Autodesk Inventor part; units mm, degrees
ref_plane "Work Plane1" through (29, 0, 0) normal (0, -1, 0) x (1, 0, 0)
ref_plane "YZ Plane" through (0, 0, 0) normal (1, 0, 0) x (0, 1, 0)
ref_plane "XZ Plane" through (0, 0, 0) normal (0, 1, 0) x (-1, 0, 0)
sketch "Sketch1" plane through (0, 0, 0) normal (0, 0, 1) x (1, 0, 0)
  line L0 (0.2, 0) -> (20, 0)
  line L1 (20, 0) -> (20, 2.5)
  line L2 (20, 2.5) -> (2.4, 2.5)
  line L3 (2.4, 2.5) -> (1.9091, 2.5)
  line L4 (1.9091, 2.5) -> (0, 2.5)
  line L5 (0, 2.5) -> (0, 4.25)
  line L6 (0, 4.25) -> (-3.5, 4.25)
  line L7 (-3.5, 4.25) -> (-3.5, 1.7321)
  line L8 (-3.5, 1.7321) -> (-0.8, 1.7321)
  line L9 (-0.8, 1.7321) -> (0.2, 0)
  line L10 (-8.2, 0) -> (24.7, 0)
  line L11 (0, -0.85) -> (0, 5.1)
  line L12 (2.4, 2.5) -> (0, 2.5) construction
  dimension "d1" = 17.6
  dimension "d2" = 0.4909
  dimension "d3" = 3.5
  dimension "d4" = 2.7
  dimension "d5" = 60
  dimension "d6" = 5
  dimension "d7" = 5
  dimension "d8" = 3.4641
  dimension "d9" = 8.5
  dimension "d26" = 20
revolve "Body" add sketch "Sketch1" angle 360 about axis through (0.2, 0, 0) along (1, 0, 0) contours L9 L11 L4 L3 L2 L1 L0 | L9 L8 L7 L6 L5 L11
sketch "Sketch2" plane through (-3.5, 0, 0) normal (-1, 0, 0) x (0, 0, 1)
  circle A0 centre (0, 0) radius 1.7321
  line L0 (0, -5.95) -> (0, 5.95)
  line L1 (-5.95, 0) -> (5.95, 0)
  line L2 (1.7321, 0) -> (0.866, -1.5)
  line L3 (0.866, -1.5) -> (-0.866, -1.5)
  line L4 (-0.866, -1.5) -> (-1.7321, 0)
  line L5 (-1.7321, 0) -> (-0.866, 1.5)
  line L6 (-0.866, 1.5) -> (0.866, 1.5)
  line L7 (0.866, 1.5) -> (1.7321, 0)
extrude "Slot" add sketch "Sketch2" against normal up to next contours L7 A0 | A0 L2 | L6 L0 A0 | A0 L0 L3 | L0 L6 A0 | A0 L3 L0 | L4 A0 | A0 L5
fillet "Fillet1" radius 0.5 1 edges at (-3.5, -4.25, 0)
thread "Thread"
chamfer "Chamfer1" distance 0.4908 distance2 0.4908 1 edges at (20, -2.5, 0) measured on face at (20, -0.7379, -0.3873)
ref_plane "Work Plane1" through (29, 0, 0) normal (0, -1, 0) x (1, 0, 0)
fillet "Fillet2" radius 0.1 1 edges at (0, -2.5, 0)
equation "\"d1\" = GEL"
equation "\"d3\" = KOH"
equation "\"d4\" = INTI"
equation "\"d6\" = GD"
equation "\"d7\" = BDM"
equation "\"d8\" = 1.1547 * SW"
equation "\"d9\" = KOD"
equation "\"d26\" = NLG"
equation "\"d30\" = R"
equation "\"d17\" = RR"
equation "\"d13\" = GEL"
equation "\"d15\" = -0.5 * SPD + 0.5 * GD"
equation "\"d16\" = GUL"
equation "\"GD\" = NND"
equation "\"NLG\" = 20"
equation "\"GEL\" = 17.6"
equation "\"KOD\" = 8.5"
equation "\"KOH\" = 3.5"
equation "\"INTI\" = 2.7"
equation "\"GAL\" = 0.61345 * PTC"
equation "\"GUL\" = 0.61345 * PTC"
equation "\"BDM\" = NND"
equation "\"SW\" = 3"
equation "\"RR\" = 0.5"
equation "\"SPD\" = NND - 1.2269 * PTC"
equation "\"R\" = 0.1"
equation "\"TOA\" = 30deg"
equation "\"GD1\" = THREADDIA - 1.2269 * PTC"
equation "\"THREADDIA\" = 5"
equation "\"FAWI\" = 45deg"
equation "\"ANG\" = 120deg"
equation "\"PTC\" = 0.8"
equation "\"NND\" = 5"
equation "\"E0\" = 1.155 * SW"
properties part number "DIN 7984 - M5 x 20" material "Steel, Mild"
CAD build for the part. Positions are in the model's coordinates, mm. A direction names the side the tool comes from. Coordinates: 2 decimals unless noted, no trailing zeros. Write each loop counter-clockwise with the first axis right and the second up, starting at its lowest first coordinate (ties: lowest second). Pieces come first, ordered by that corner, then holes. Notation, with made-up numbers: (66.5, 46.5) -> (104.5, 46.5) arc R17 ccw to (104.5, 74.5) -> close; hole circle Ø7 at (-29.75, -24.75). An arc over 180 degrees is marked (long way). Return JSON: item names as keys, results as strings. Group by question number.
Q1. Pull direction Z, two halves, no side cores. Call faces 4 (the face through (20, 0, 0)), 5 (the face through (-1.521, 2.285, -3.584)), 6 (the face through (-2, 1.5, 0)): released by +Z, released by -Z, zero draft, split by the parting line, or undercut.
Q2. Flat gauge pins, fed straight in: pin 1 (4 mm diameter, centred on x = 16.5, z = -3, fed in from +Y); pin 2 (4 mm diameter, centred on x = 6.5, z = -3.5, fed in from -Y); pin 3 (5 mm diameter, centred on x = 3, y = -3, fed in from +Z). Where does each tip first touch, or does it go through?
Q3. Which spindle directions (+Z, -Z, +X, -X, +Y, -Y) get a long thin tool onto all of the face, cutting with end or side? Do faces 1 (the face through (0, 2, 2)), 2 (the face through (-3.5, -2, 0)), 3 (the face through (-2, -1.5, 0)). Say none if no direction does.
Q4. Drill centre lines: line 1 (X direction, y = 2.25, z = -2.75); line 2 (Z direction, x = -1.5, y = 1.25); line 3 (Z direction, x = 5, y = 2). Where is each one in solid material? Low to high.
Q5. Cut at A-A, the plane x = 9.5. Give the cut face in (y, z), then the cut area to 3 significant figures.
Returned:
{
 "1": {"face 4": "zero draft", "face 5": "split by the parting line", "face 6": "undercut"},
 "2": {"pin 1": "stops at y = 2.29", "pin 2": "stops at y = -2", "pin 3": "stops at z = 2.45"},
 "3": {"face 1": "+X", "face 2": "+Z, -Z, -X, +Y, -Y", "face 3": "-X"},
 "4": {"line 1": "x = -3.5 to 0", "line 2": "z = -4.06 to -1.01, 1.01 to 4.06", "line 3": "z = -1.5 to 1.5"},
 "5": {"outline": "circle Ø5 at (0, 0)", "area": "19.6 mm2"}
}
